```python
from build123d import *

# Parameters (mm, degrees)
SKETCH1_R           = 1.6
SKETCH1_R_2         = 6
BOSS_EXTRUDE1_DEPTH = 3


with BuildPart() as part:
    # Sketch1 → Boss-Extrude1 (new body)
    with BuildSketch(Plane.XY):
        with BuildLine():
            ThreePointArc((13.513146708, -41.545306592), (16.804211194, -46.236480195), (20.095275679, -41.545306592))
            ThreePointArc((20.095275679, -41.545306592), (20.125665024, -40.105234948), (21.115730483, -39.059051292))
            ThreePointArc((21.115730483, -39.059051292), (23.892956675, -37.097303615), (25.854704352, -34.320077422))
            ThreePointArc((25.854704352, -34.320077422), (26.900888008, -33.330011964), (28.340959652, -33.299622619))
            ThreePointArc((28.340959652, -33.299622619), (33.032133255, -30.008558133), (28.340959652, -26.717493648))
            ThreePointArc((28.340959652, -26.717493648), (26.900888008, -26.687104303), (25.854704352, -25.697038844))
            ThreePointArc((25.854704352, -25.697038844), (23.892956675, -22.919812652), (21.115730483, -20.958064974))
            ThreePointArc((21.115730483, -20.958064974), (20.125665024, -19.911881319), (20.095275679, -18.471809674))
            ThreePointArc((20.095275679, -18.471809674), (16.804211194, -13.780636072), (13.513146708, -18.471809674))
            ThreePointArc((13.513146708, -18.471809674), (13.482757363, -19.911881319), (12.492691904, -20.958064974))
            ThreePointArc((12.492691904, -20.958064974), (6.779211194, -30.008558133), (12.492691904, -39.059051292))
            ThreePointArc((12.492691904, -39.059051292), (13.482757363, -40.105234948), (13.513146708, -41.545306592))
        make_face()
        with Locations((16.804211194, -17.280636072)):
            Circle(SKETCH1_R, mode=Mode.SUBTRACT)
        with Locations((16.804211194, -30.008558133)):
            Circle(SKETCH1_R_2, mode=Mode.SUBTRACT)
        with Locations((16.804211194, -42.736480195)):
            Circle(SKETCH1_R, mode=Mode.SUBTRACT)
        with Locations((29.532133255, -30.008558133)):
            Circle(SKETCH1_R, mode=Mode.SUBTRACT)
    extrude(amount=BOSS_EXTRUDE1_DEPTH)


solid = part.part
```
Can you work these out from the model? Positions are in its coordinate system, mm. Give positions to 0.01 mm unless a question says otherwise; leave off trailing zeros. Loops run counter-clockwise (first coordinate to the right, second up) from the corner with the lowest first, then second, coordinate; pieces in that order, holes last. Notation, with made-up numbers: M -0.5,43.5 L 7.5,43.5 A30 cw 7.5,75.5 Z; hole C 5.5,60 d1. An arc over 180 degrees is marked long. One line per item, written item: value.
(1) Suppose I cut it at C-C on z = 1.35. Count the separate pieces of the cut face and the enclosed holes in it, plus the area to 3 significant figures.
Returned:
separate pieces: 1
enclosed holes: 4
area: 295 mm^2
(2) Suppose I cut it at B-B on x = 18. List the corners of the cut face in (y, z) for me.
Returned:
outline: M -46.03,0 L -43.8,0 L -43.8,3 L -46.03,3 Z; M -41.67,0 L -35.89,0 L -35.89,3 L -41.67,3 Z; M -24.13,0 L -18.34,0 L -18.34,3 L -24.13,3 Z; M -16.22,0 L -13.99,0 L -13.99,3 L -16.22,3 Z
(3) I need wall thicknesses on line 1 (Y direction, x = 15.75, z = 1.5); line 2 (Y direction, x = 17, z = 0.9); line 3 (Y direction, x = 14.5, z = 1.6). Which ranges of each line are inside material? Lowest first, please.
Returned:
line 1: -46.07 to -43.94, -41.53 to -35.92, -24.1 to -18.48, -16.08 to -13.94
line 2: -46.23 to -44.32, -41.15 to -36.01, -24.01 to -18.87, -15.69 to -13.79
line 3: -45.37 to -35.55, -24.47 to -14.65
(4) We'd pull the mould along Y, two halves only. Please class faces 1 (the face through (26.92, -26.695, 1.479)), 2 (the face through (33.03, -30.1, 1.48)), 3 (the face through (13.49, -19.89, 1.48)): released by +Y, released by -Y, zero draft, split by the parting line, or undercut.
Returned:
face 1: released by +Y
face 2: split by the parting line
face 3: undercut
(5) Will these pins go through, and if not, where does the flat tip stop? pin 1 (1.5 mm diameter, centred on x = 26.5, z = 1, fed in from +Y); pin 2 (1 mm diameter, centred on x = 25.5, z = 1.5, fed in from -Y).
Returned:
pin 1: y = -25.48
pin 2: y = -35.78
(6) Suppose I cut it at D-D on x = 11.5. List the corners of the cut face in (y, z) for me, plus the area to 3 significant figures.
Returned:
outline: M -38.52,0 L -32.81,0 L -32.81,3 L -38.52,3 Z; M -27.2,0 L -21.5,0 L -21.5,3 L -27.2,3 Z
area: 34.2 mm^2
(7) Suppose I cut it at A-A on y = -18. List the corners of the cut face in (x, z) for me, plus the area to 3 significant figures.
Returned:
outline: M 13.38,0 L 15.38,0 L 15.38,3 L 13.38,3 Z; M 18.23,0 L 20.23,0 L 20.23,3 L 18.23,3 Z
area: 12.0 mm^2
